Read the model definition and answer for the solid it produces. Units are mm, in the model's axes. A direction names the side the tool comes from. Round coordinates to 2 decimals unless told otherwise and drop trailing zeros. Order: outer loops, then holes, each group sorted by start corner. A loop starts at its lowest first (then second) coordinate and runs counter-clockwise, first axis right, second up. Notation, with made-up numbers: (-1, 83.5) -> (29, 83.5) arc R17 cw to (29, 108.5) -> close; hole circle Ø10 at (16, -17). An arc over 180 degrees is marked (long way). Answer as a JSON object with one key per item and string values. Group by question number.
Item 1: Given P1, Ø2, axis at y = 3, z = -32.5, coming from the +X side; P2, Ø2, axis at y = 2, z = -188, coming from the -X side; P3, Ø1.2, axis at x = 10.5, y = 2, coming from the +Z side; P4, Ø3, axis at x = 5, z = -125, coming from the +Y side, each flat-ended and moving along its own axis, determine where each tip first touches the part or whether it passes through.
Item 2: The mould has two halves that part along X. Classify faces 5 (the flat face through (30, 2, -195)), 6 (the cylindrical face through (4.06, 2.03, -126.23)), 7 (the flat face through (32, 0, -126)): pulls with the +X half, pulls with the -X half, needs draft (parallel to the pull), parting line crosses it, or undercut.
Item 3: Section C-C, the plane y = 2.95 is taken. Write down the section's boundary in (x, z).
Item 4: Section A-A, the plane x = 40 is taken. Write down the section's boundary in (y, z), plus the area to 3 significant figures.
Item 5: Section D-D, the plane z = -99 is taken. Write down the section's boundary in (x, y), plus the area to 3 significant figures.
Item 6: For faces 1 (the flat face through (52, 2, -204)), 2 (the flat face through (50, 2, -218)), 3 (the flat face through (15, 2, -170)), 4 (the flat face through (50, 2, -32)), determine the directions among +Z, -Z, +X, -X, +Y, -Y from which every point of the face is accessible in a straight line to the end or side of a thin tool.
Item 7: Section B-B, the plane z = -210 is taken. Write down the section's boundary in (x, y), plus the area to 3 significant figures.
Item 8: Consider probe 1 along X at (y, z) = (1.05, -135); probe 2 along X at (y, z) = (1.2, -125); probe 3 along Z at (x, y) = (42, 0.75). Determine where each line is inside the solid, lowest interval first. Write a range as from..to.
from build123d import *

# Parameters (mm, degrees)
CROQUIS1_W              = 250
CROQUIS1_H              = 250
CROQUIS1_R              = 2.5
SALIENTE_EXTRUIR1_DEPTH = 4
CORTAR_EXTRUIR1_DEPTH   = 4
CROQUIS3_W              = 150
CROQUIS3_H              = 150
CROQUIS3_W_2            = 100
CROQUIS3_H_2            = 100
SALIENTE_EXTRUIR2_DEPTH = 4
CROQUIS4_R              = 1.55
CORTAR_EXTRUIR2_DEPTH   = 10
CROQUIS5_W              = 150
CROQUIS5_H              = 150
CROQUIS5_W_2            = 100
CROQUIS5_H_2            = 100
CORTAR_EXTRUIR3_DEPTH   = 10
CROQUIS6_W              = 30
CROQUIS6_H              = 50
CROQUIS6_W_2            = 50
CROQUIS6_H_2            = 30
CORTAR_EXTRUIR4_DEPTH   = 10
CROQUIS8_R              = 1.55
CORTAR_EXTRUIR5_DEPTH   = 10
CORTAR_EXTRUIR6_DEPTH   = 10


with BuildPart() as part:
    # Croquis1 → Saliente-Extruir1 (new body)
    with BuildSketch(Plane(origin=(0, 0, 0), x_dir=(1, 0, 0), z_dir=(0, 1, 0))):
        with Locations((125, 125)):
            Rectangle(CROQUIS1_W, CROQUIS1_H)
        with Locations(Location((40, 210, 0), (0, 0, 270))):
            Circle(CROQUIS1_R, mode=Mode.SUBTRACT)
        with Locations(Location((210, 210, 0), (0, 0, 270))):
            Circle(CROQUIS1_R, mode=Mode.SUBTRACT)
        with Locations(Location((210, 40, 0), (0, 0, 270))):
            Circle(CROQUIS1_R, mode=Mode.SUBTRACT)
        with Locations(Location((40, 40, 0), (0, 0, 270))):
            Circle(CROQUIS1_R, mode=Mode.SUBTRACT)
    extrude(amount=SALIENTE_EXTRUIR1_DEPTH)

    # Croquis2 → Cortar-Extruir1 (cut)
    with BuildSketch(Plane(origin=(0, 4, 0), x_dir=(1, 0, 0), z_dir=(0, 1, 0))):
        Polygon((50, 50), (200, 50), (200, 200), (50, 200), (50, 150.09044268), align=None)
    extrude(amount=-CORTAR_EXTRUIR1_DEPTH, mode=Mode.SUBTRACT)

    # Croquis3 → Saliente-Extruir2 (add)
    with BuildSketch(Plane(origin=(0, 4, 0), x_dir=(1, 0, 0), z_dir=(0, 1, 0))):
        with Locations((125, 125)):
            Rectangle(CROQUIS3_W, CROQUIS3_H)
        with Locations((125, 125)):
            Rectangle(CROQUIS3_W_2, CROQUIS3_H_2, mode=Mode.SUBTRACT)
    extrude(amount=-SALIENTE_EXTRUIR2_DEPTH)

    # Croquis4 → Cortar-Extruir2 (cut)
    with BuildSketch(Plane(origin=(0, 4, 0), x_dir=(1, 0, 0), z_dir=(0, 1, 0))):
        with Locations(Location((115, 20, 0), (0, 0, 270))):
            Circle(CROQUIS4_R)
        with Locations(Location((135, 20, 0), (0, 0, 270))):
            Circle(CROQUIS4_R)
        with Locations(Location((125, 5, 0), (0, 0, 270))):
            Circle(CROQUIS4_R)
    extrude(amount=-CORTAR_EXTRUIR2_DEPTH, mode=Mode.SUBTRACT)

    # Croquis5 → Cortar-Extruir3 (cut)
    with BuildSketch(Plane(origin=(0, 4, 0), x_dir=(1, 0, 0), z_dir=(0, 1, 0))):
        with Locations((125, 125)):
            Rectangle(CROQUIS5_W, CROQUIS5_H)
        with Locations((125, 125)):
            Rectangle(CROQUIS5_W_2, CROQUIS5_H_2, mode=Mode.SUBTRACT)
    extrude(amount=-CORTAR_EXTRUIR3_DEPTH, mode=Mode.SUBTRACT)

    # Croquis6 → Cortar-Extruir4 (cut)
    with BuildSketch(Plane(origin=(0, 4, 0), x_dir=(1, 0, 0), z_dir=(0, 1, 0))):
        Polygon((170, 0), (250, 0), (250, 30), (220, 30), (170, 30), align=None)
        with Locations((235, 55)):
            Rectangle(CROQUIS6_W, CROQUIS6_H)
        Polygon((0, 80), (0, 0), (30, 0), (30, 30), (30, 80), align=None)
        with Locations((55, 15)):
            Rectangle(CROQUIS6_W_2, CROQUIS6_H_2)
        Polygon((80, 250), (0, 250), (0, 220), (30, 220), (80, 220), align=None)
        with Locations((15, 195)):
            Rectangle(CROQUIS6_W, CROQUIS6_H)
        Polygon((250, 170), (250, 250), (220, 250), (220, 220), (220, 170), align=None)
        with Locations((195, 235)):
            Rectangle(CROQUIS6_W_2, CROQUIS6_H_2)
    extrude(amount=-CORTAR_EXTRUIR4_DEPTH, mode=Mode.SUBTRACT)

    # Croquis8 → Cortar-Extruir5 (cut)
    with BuildSketch(Plane(origin=(0, 4, 0), x_dir=(1, 0, 0), z_dir=(0, 1, 0))):
        with Locations(Location((125, 5, 0), (0, 0, 270))):
            Circle(CROQUIS8_R)
        with Locations(Location((135, 20, 0), (0, 0, 270))):
            Circle(CROQUIS8_R)
        with Locations(Location((115, 20, 0), (0, 0, 270))):
            Circle(CROQUIS8_R)
        with Locations(Location((20, 135, 0), (0, 0, 270))):
            Circle(CROQUIS8_R)
        with Locations(Location((5, 125, 0), (0, 0, 270))):
            Circle(CROQUIS8_R)
        with Locations(Location((20, 115, 0), (0, 0, 270))):
            Circle(CROQUIS8_R)
        with Locations(Location((135, 230, 0), (0, 0, 270))):
            Circle(CROQUIS8_R)
        with Locations(Location((125, 245, 0), (0, 0, 270))):
            Circle(CROQUIS8_R)
        with Locations(Location((115, 230, 0), (0, 0, 270))):
            Circle(CROQUIS8_R)
        with Locations(Location((230, 115, 0), (0, 0, 270))):
            Circle(CROQUIS8_R)
        with Locations(Location((245, 125, 0), (0, 0, 270))):
            Circle(CROQUIS8_R)
        with Locations(Location((230, 135, 0), (0, 0, 270))):
            Circle(CROQUIS8_R)
    extrude(amount=-CORTAR_EXTRUIR5_DEPTH, mode=Mode.SUBTRACT)

    # Croquis9 → Cortar-Extruir6 (cut)
    with BuildSketch(Plane(origin=(0, 4, 0), x_dir=(1, 0, 0), z_dir=(0, 1, 0))):
        Polygon((50, 0), (250, 0), (250, 250), (50, 250), (50, 216), (53, 216), (53, 204), (50, 204), (50, 46), (53, 46), (53, 34), (50, 34), align=None)
    extrude(amount=-CORTAR_EXTRUIR6_DEPTH, mode=Mode.SUBTRACT)


solid = part.part
Values found:
{
 "1": {"P1": "x = 50", "P2": "x = 30", "P3": "z = -80", "P4": "through"},
 "2": {"face 5": "pulls with the -X half", "face 6": "undercut", "face 7": "needs draft"},
 "3": {"outline": "(0, -170) -> (30, -170) -> (30, -220) -> (50, -220) -> (50, -216) -> (53, -216) -> (53, -204) -> (50, -204) -> (50, -46) -> (53, -46) -> (53, -34) -> (50, -34) -> (50, -30) -> (30, -30) -> (30, -80) -> (0, -80) -> close; hole circle Ø3.1 at (5, -125); hole circle Ø3.1 at (20, -135); hole circle Ø3.1 at (20, -115); hole circle Ø5 at (40, -210); hole circle Ø5 at (40, -40)"},
 "4": {"outline": "(0, -220) -> (4, -220) -> (4, -212.5) -> (0, -212.5) -> close; (0, -207.5) -> (4, -207.5) -> (4, -42.5) -> (0, -42.5) -> close; (0, -37.5) -> (4, -37.5) -> (4, -30) -> (0, -30) -> close", "area": "720 mm2"},
 "5": {"outline": "(0, 0) -> (50, 0) -> (50, 4) -> (0, 4) -> close", "area": "200 mm2"},
 "6": {"face 1": "+X, +Y, -Y", "face 2": "-Z, +X, +Y, -Y", "face 3": "-Z, -X, +Y, -Y", "face 4": "+Z, +X, +Y, -Y"},
 "7": {"outline": "(30, 0) -> (37.5, 0) -> (37.5, 4) -> (30, 4) -> close; (42.5, 0) -> (53, 0) -> (53, 4) -> (42.5, 4) -> close", "area": "72.0 mm2"},
 "8": {"probe 1": "0..18.45, 21.55..50", "probe 2": "0..3.45, 6.55..50", "probe 3": "-220..-211.5, -208.5..-41.5, -38.5..-30"}
}
